Autodesk Inventor part; units mm, degrees
ref_plane "mitCover_XY" through (0, 0, 0) normal (0, 1, 0) x (1, 0, 0)
ref_plane "mitCover_YZ" through (0, 0, 0) normal (1, 0, 0) x (0, 0, -1)
ref_plane "mitCover_ZX" through (0, 0, 0) normal (0, 0, -1) x (0, 1, 0)
sketch "Sketch_1" plane through (0, 0, 0) normal (1, 0, 0) x (0, 1, 0)
  line L0 (0.8, 3.9) -> (0, 3.9)
  line L1 (0, 3.9) -> (0, -3.9)
  line L2 (0, -3.9) -> (0.8, -3.9)
  arc A0 (0.8, -3.9) -> (1, -3.7) centre (0.8, -3.7) ccw
  line L3 (1, -3.7) -> (1, 3.7)
  arc A1 (1, 3.7) -> (0.8, 3.9) centre (0.8, 3.7) ccw
extrude "Extrusion1" add sketch "Sketch_1" along normal mid plane 13.3
sketch "Sketch_2" plane through (0, 0, 0) normal (0, 0, 1) x (1, 0, 0)
  line L0 (5, -1.7) -> (5, 0)
  line L1 (5, 0) -> (5.5, 0)
  line L2 (5.5, 0) -> (5.5, -1.7)
  line L3 (5.5, -1.7) -> (5, -1.7)
  line L4 (5, -1.7) -> (5, 0)
revolve "Revolution1" add sketch "Sketch_2" angle 360 about axis through (5, -1.7, 0) along (0, -1, 0)
sketch "Sketch_3" plane through (0, 0, 0) normal (0, 0, 1) x (1, 0, 0)
  line L0 (-5, -1.7) -> (-5, 0)
  line L1 (-5, 0) -> (-4.5, 0)
  line L2 (-4.5, 0) -> (-4.5, -1.7)
  line L3 (-4.5, -1.7) -> (-5, -1.7)
  line L4 (-5, -1.7) -> (-5, 0)
revolve "Revolution2" add sketch "Sketch_3" angle 360 about axis through (-5, -1.7, 0) along (0, -1, 0)
ref_plane "mitCover_XY" through (0, 0, 0) normal (0, 1, 0) x (1, 0, 0)
ref_plane "mitCover_YZ" through (0, 0, 0) normal (1, 0, 0) x (0, 0, -1)
ref_plane "mitCover_ZX" through (0, 0, 0) normal (0, 0, -1) x (0, 1, 0)
properties part number "ESG 8x13.5 1912130000"
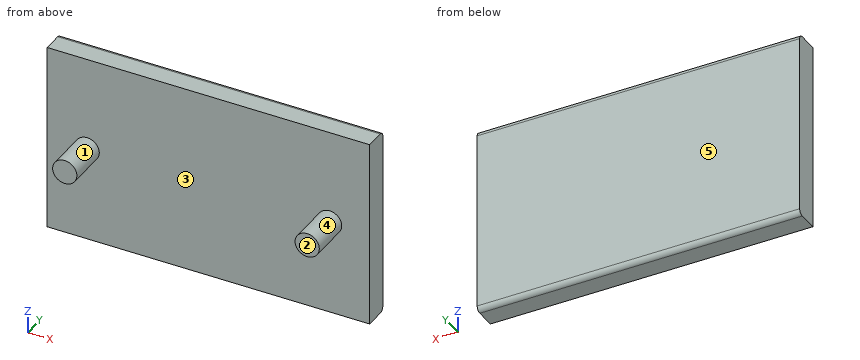
Verification items for the finished model (mm, model axes). Face numbers are marked on the shaded views. A direction names the side the tool comes from. Give positions to 0.01 mm unless a question says otherwise; leave off trailing zeros. Order: outer loops, then holes, each group sorted by start corner. A loop starts at its lowest first (then second) coordinate and runs counter-clockwise, first axis right, second up. Notation, with made-up numbers: M 67,71 L 102,71 A25 ccw 102,95 Z; hole C 35.25,16.25 d11. An arc over 180 degrees is marked long. Use one line per item in the form item = value. Start each with the question number.
Q1. Go/stop test with a flat-tipped pin: pin 1 Ø3 at (x, z) = (-0.5, 2.5) entering from -Y. Record where the tip stops, or that it passes through.
Q2. Section check D-D (z = -2.5). Enter the section's corners in (x, y), then the cut area to 3 significant figures.
Q3. Scan lines: line 1 along Y through (x, z) = (-2, 3.5); line 2 along X through (y, z) = (-0.05, -0.25); line 3 along Z through (x, y) = (-3.5, 0.85). Record each from-to range of solid material in increasing order. Write a range as [from, to].
Q4. Section check B-B (y = -0.6). Enter the section's corners in (x, z).
Q5. Section check C-C (x = -1.75). Enter the section's corners in (y, z), then the cut area to 3 significant figures.
Q6. Access from +Z, -Z, +X, -X, +Y, -Y to the whole of each face (thin tool, end or side, straight path). Record for the marked faces 1 and 2.
Q7. Mould release check, pull along Y, two halves, no side actions. Record for the marked faces 3, 4 and 5: +Y half, -Y half, draft (parallel to the pull), parting line (faces both ways), or undercut.
Q8. Section check A-A (x = -5). Enter the section's corners in (y, z), then the cut area to 3 significant figures.
Evaluation:
q1.pin_1 = 0
q2.outline = M -6.65,0 L 6.65,0 L 6.65,1 L -6.65,1 Z
q2.area = 13.3 mm2
q3.line_1 = [0, 1]
q3.line_2 = [-5.43, -4.57], [4.57, 5.43]
q3.line_3 = [-3.89, 3.89]
q4.outline = C -5,0 d1; C 5,0 d1
q5.outline = M 0,-3.9 L 0.8,-3.9 A0.2 ccw 1,-3.7 L 1,3.7 A0.2 ccw 0.8,3.9 L 0,3.9 Z
q5.area = 7.78 mm2
q6.face_1 = -Y
q6.face_2 = +Z, -Z, +X, -X, -Y
q7.face_3 = -Y half
q7.face_4 = draft
q7.face_5 = +Y half
q8.outline = M -1.7,-0.5 L 0,-0.5 L 0,-3.9 L 0.8,-3.9 A0.2 ccw 1,-3.7 L 1,3.7 A0.2 ccw 0.8,3.9 L 0,3.9 L 0,0.5 L -1.7,0.5 Z
q8.area = 9.48 mm2
